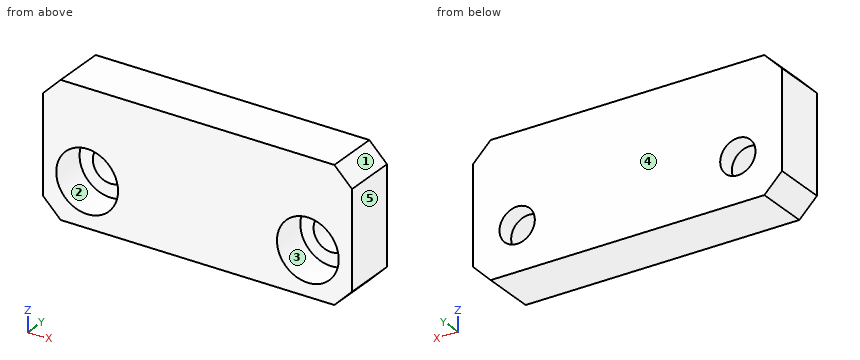
```python
from build123d import *

# Parameters (mm, degrees)
F0_W     = 35
F0_H     = 15
F1_DEPTH = 6
F2_R     = 3.5
F3_DEPTH = 4
F4_R     = 2
F5_DEPTH = 6.001
F6_SIZE  = 2


with BuildPart() as f1:
    # F0 (on Front) → F1 (new body)
    with BuildSketch(Plane.XZ):
        Rectangle(F0_W, F0_H)
    extrude(amount=F1_DEPTH)

    # F2 (on face) → F3 (cut)
    with BuildSketch(Plane.XZ.offset(6)):
        with Locations((12.5, -2.5)):
            Circle(F2_R)
        with Locations((-12.5, -2.5)):
            Circle(F2_R)
    extrude(amount=-F3_DEPTH, mode=Mode.SUBTRACT)

    # F4 (on face) → F5 (cut, through all)
    with BuildSketch(Plane.XZ.offset(6)):
        with Locations((12.5, -2.5)):
            Circle(F4_R)
        with Locations((-12.5, -2.5)):
            Circle(F4_R)
    extrude(amount=-F5_DEPTH, mode=Mode.SUBTRACT)

    # F6
    f6_edges = [f1.edges().sort_by_distance(p)[0] for p in [
        (-17.5, -3, 7.5),
        (17.5, -3, 7.5),
        (17.5, -3, -7.5),
        (-17.5, -3, -7.5),
    ]]
    chamfer(f6_edges, length=F6_SIZE)


solid = f1.part
```
Check sheet for the modelled part. Datum: model origin and axes. Units: mm. Face numbers are marked on the shaded views. A direction names the side the tool comes from. Coordinates: 2 decimals unless noted, no trailing zeros. Loops run counter-clockwise (first coordinate to the right, second up) from the corner with the lowest first, then second, coordinate; pieces in that order, holes last.
1) Sectioned sample at A-A (z = -2.5). Record the boundary of the cut face in (x, y), and give its area (3 significant figures).
2) Material ranges on probe 1 along Z at (x, y) = (12.5, -0.35); probe 2 along Z at (x, y) = (12.5, -3.2); probe 3 along Y at (x, z) = (12, -0.5), recorded low to high.
3) Gauge pin test, flat end, axial feed: pin 1 (3.5 mm diameter, centred on x = 11, z = -2, fed in from -Y). Record the tip position at first contact, or that the pin passes through.
4) Access from +Z, -Z, +X, -X, +Y, -Y to the whole of each face (thin tool, end or side, straight path). Record for the marked faces 1 and 2.
5) Sectioned sample at B-B (x = -12.5). Record the boundary of the cut face in (y, z), and give its area (3 significant figures).
6) Release check for a two-part mould opening along X. For the marked faces 3, 4 and 5 record: released by +X, released by -X, zero draft, split by the parting line, or undercut.
7) Sectioned sample at C-C (y = -3.15). Record the boundary of the cut face in (x, z).
8) Sectioned sample at D-D (x = 10). Record the boundary of the cut face in (y, z), and give its area (3 significant figures).
Check sheet entries:
1. outline: (-17.5, -6) - (-16, -6) - (-16, -2) - (-14.5, -2) - (-14.5, 0) - (-17.5, 0) - close; (-10.5, -2) - (-9, -2) - (-9, -6) - (9, -6) - (9, -2) - (10.5, -2) - (10.5, 0) - (-10.5, 0) - close; (14.5, -2) - (16, -2) - (16, -6) - (17.5, -6) - (17.5, 0) - (14.5, 0) - close
1. area: 138 mm2
2. probe 1: z = -7.5 to -4.5, -0.5 to 7.5
2. probe 2: z = -7.5 to -6, 1 to 7.5
2. probe 3: y = -2 to 0
3. pin 1: stops at y = -2
4. face 1: +Z, +X, +Y, -Y
4. face 2: -Y
5. outline: (-6, -7.5) - (0, -7.5) - (0, -4.5) - (-2, -4.5) - (-2, -6) - (-6, -6) - close; (-6, 1) - (-2, 1) - (-2, -0.5) - (0, -0.5) - (0, 7.5) - (-6, 7.5) - close
5. area: 54.0 mm2
6. face 3: undercut
6. face 4: zero draft
6. face 5: released by +X
7. outline: (-17.5, -5.5) - (-15.5, -7.5) - (15.5, -7.5) - (17.5, -5.5) - (17.5, 5.5) - (15.5, 7.5) - (-15.5, 7.5) - (-17.5, 5.5) - close; hole circle Ø7 at (-12.5, -2.5); hole circle Ø7 at (12.5, -2.5)
8. outline: (-6, -7.5) - (0, -7.5) - (0, 7.5) - (-6, 7.5) - (-6, -0.05) - (-2, -0.05) - (-2, -4.95) - (-6, -4.95) - close
8. area: 70.4 mm2
